```python
from build123d import *

# Parameters (mm, degrees)
BOSS_EXTRUDE1_DEPTH = 3
FILLET1_R           = 4
FILLET2_R           = 1
FILLET3_R           = 1


with BuildPart() as part:
    # Sketch1 → Boss-Extrude1 (new body)
    with BuildSketch(Plane.XY):
        with BuildLine():
            Line((0, 43.376726626), (0, 37.5))
            ThreePointArc((0, 37.5), (-36.914491769, 6.600780063), (-12.99543687, -35.176250803))
            Line((-12.99543687, -35.176250803), (-6.107994139, -47.105651546))
            ThreePointArc((-6.107994139, -47.105651546), (-47.401310364, 3.060355499), (0, 47.5))
            Line((0, 47.5), (0, 52.5))
            Line((0, 52.5), (6.75, 52.5))
            Line((6.75, 52.5), (6.75, 37.5))
            Line((6.75, 37.5), (1.79, 37.5))
            Line((1.79, 37.5), (1.79, 43.376726626))
            Line((1.79, 43.376726626), (0, 43.376726626))
        make_face()
    extrude(amount=BOSS_EXTRUDE1_DEPTH)

    # Fillet1
    fillet1_edges = [part.edges().sort_by_distance(p)[0] for p in [
        (0, 47.5, 1.5),
    ]]
    fillet(fillet1_edges, radius=FILLET1_R)

    # Fillet2
    fillet2_edges = [part.edges().sort_by_distance(p)[0] for p in [
        (-12.99543687, -35.176250803, 1.5),
    ]]
    fillet(fillet2_edges, radius=FILLET2_R)

    # Fillet3
    fillet3_edges = [part.edges().sort_by_distance(p)[0] for p in [
        (-6.107994139, -47.105651546, 1.5),
    ]]
    fillet(fillet3_edges, radius=FILLET3_R)


solid = part.part
```
Could you check a few things on this model? Use its own coordinates, in mm. A direction names the side the tool comes from. Give positions to 0.01 mm unless a question says otherwise; leave off trailing zeros. Order: outer loops, then holes, each group sorted by start corner. A loop starts at its lowest first (then second) coordinate and runs counter-clockwise, first axis right, second up.
Q1. We'd pull the mould along Y, two halves only. Please class faces 4 (the cylindrical face through (-36.744, 7.491, 1.479)), 5 (the flat face through (4, 37.5, 1)), 6 (the flat face through (6.75, 45, 1)): +Y half, -Y half, draft (parallel to the pull), parting line (faces both ways), or undercut.
Q2. Suppose I cut it at A-A, the plane z = 0.6. Write out the boundary of the cut face in (x, y), and give its area (3 significant figures).
Q3. If I drill on line 1 along Y through (x, z) = (2.5, 2.75); line 2 along X through (y, z) = (-1, 1.3); line 3 along Y through (x, z) = (-25, 0.5), over which ranges is the centre line in solid material (lowest first)?
Q4. For faces 1 (the flat face through (-10.02, -40.33, 1.48)), 2 (the flat face through (1, 43.377, 1)), 3 (the flat face through (3, 52.5, 1)), which set-ups out of +Z, -Z, +X, -X, +Y, -Y let a thin tool reach every point of the face, with its end or its side?
Q5. Suppose I cut it at C-C, the plane y = 41. Write out the boundary of the cut face in (x, z), and give its area (3 significant figures).
Q6. Suppose I cut it at B-B, the plane x = -24. Write out the boundary of the cut face in (y, z).
Q7. Suppose I cut it at D-D, the plane x = -1.5. Write out the boundary of the cut face in (y, z), and give its area (3 significant figures).
Q8. I'm going to push flat-ended pins straight in: P1, Ø0.9, axis at y = 41, z = 1, coming from the -X side; P2, Ø1.5, axis at y = -33.5, z = 1.5, coming from the +X side; P3, Ø0.9, axis at y = 52, z = 1, coming from the -X side. Where does each tip first touch, or does it pass through?
Solution:
1. face 4: undercut
1. face 5: -Y half
1. face 6: draft
2. outline: (-13.33, -35.05) arc R37.5 cw to (0, 37.5) - (0, 43.38) - (1.79, 43.38) - (1.79, 37.5) - (6.75, 37.5) - (6.75, 52.5) - (0, 52.5) - (0, 51.34) arc R4 cw to (-3.69, 47.36) arc R47.5 ccw to (-8.19, -46.79) arc R1 ccw to (-7.15, -45.3) - (-12.82, -35.49) arc R1 ccw to start
2. area: 1,330 mm2
3. line 1: y = 37.5 to 52.5
3. line 2: x = -47.49 to -37.49
3. line 3: y = -40.39 to -27.95, 27.95 to 40.39
4. face 1: +Z, -Z, +X
4. face 2: +Z, -Z, -Y
4. face 3: +Z, -Z, +X, -X, +Y
5. outline: (-23.98, 0) - (0, 0) - (0, 3) - (-23.98, 3) - close; (1.79, 0) - (6.75, 0) - (6.75, 3) - (1.79, 3) - close
5. area: 86.8 mm2
6. outline: (-40.99, 0) - (-28.81, 0) - (-28.81, 3) - (-40.99, 3) - close; (28.81, 0) - (40.99, 0) - (40.99, 3) - (28.81, 3) - close
7. outline: (37.47, 0) - (48.22, 0) - (48.22, 3) - (37.47, 3) - close
7. area: 32.3 mm2
8. P1: stops at x = -24.74
8. P2: stops at x = -15.27
8. P3: stops at x = 0
